```python
from build123d import *

# Parameters (mm, degrees)
SKETCH1_W                     = 312.66
SKETCH1_H                     = 183.16
BODY_DEPTH                    = 4.7
F_6_32_TAPPED_HOLE1_D         = 2.7051
RISER_CABLE_CUTOUT_REACH      = 364.389
EXPANSION_CUTOUT_REACH        = 364.389
SKETCH11_W                    = 138.78
SKETCH11_H                    = 61.66
PSU_CABLE_CUTOUT_REACH        = 364.389
SKETCH20_W                    = 45
SKETCH20_H                    = 15
SSD_ACCESS_CUTOUT_REACH       = 364.389
SKETCH22_W                    = 123.78
SKETCH22_H                    = 72
TAP_DRILL_FOR_M3X0_5_TAP1_D   = 2.5
HOLE_IN_STOCK_REACH           = 364.389
SKETCH33_W                    = 173.88
SKETCH33_H                    = 23.33
BOSS_EXTRUDE1_DEPTH           = 1.5
TAP_DRILL_FOR_6_32_TAP1_D     = 2.7051
TAP_DRILL_FOR_6_32_TAP1_DEPTH = 15.24
TAP_DRILL_FOR_6_32_TAP1_TIP   = 0.81269403
SKETCH32_W                    = 119.186565276
SKETCH32_H                    = 183.16
CUT_EXTRUDE1_DEPTH            = 2


with BuildPart() as part:
    # Sketch1 → body (new body)
    with BuildSketch(Plane(origin=(0, 0, 0), x_dir=(0, 0, -1), z_dir=(1, 0, 0))):
        with Locations((-156.33, 91.58)):
            Rectangle(SKETCH1_W, SKETCH1_H)
    extrude(amount=BODY_DEPTH)

    # #6-32 Tapped Hole1 (through all)
    with Locations(Plane(origin=(4.7, 169.81, 166.8), x_dir=(0, 0, 1), z_dir=(1, 0, 0))):
        with Locations((0, 0), (-154.94, 0), (-132.08, 157.48), (0, 157.48)):
            Hole(F_6_32_TAPPED_HOLE1_D / 2)

    # Sketch8 → riser-cable-cutout (cut, up to next)
    with BuildSketch(Plane(origin=(4.7, 0, 0), x_dir=(0, 0, -1), z_dir=(1, 0, 0)), mode=Mode.PRIVATE) as riser_cable_cutout_sk1:
        Polygon((-148.58070669, 183.16), (-20.810027071, 183.16), (-20.810027071, 176.16), (-20.810027071, 168.16), (-148.58070669, 168.16), (-148.58070669, 176.16), align=None)
    riser_cable_cutout_tool1 = extrude(riser_cable_cutout_sk1.sketch, amount=-RISER_CABLE_CUTOUT_REACH, mode=Mode.PRIVATE) & part.part
    add(riser_cable_cutout_tool1.solids().sort_by_distance((4.7, 175.66, 84.695367))[0], mode=Mode.SUBTRACT)

    # Sketch11 → expansion-cutout (cut, up to next)
    with BuildSketch(Plane(origin=(4.7, 0, 0), x_dir=(0, 0, -1), z_dir=(1, 0, 0)), mode=Mode.PRIVATE) as expansion_cutout_sk1:
        with Locations((-243.27, 30.83)):
            Rectangle(SKETCH11_W, SKETCH11_H)
    expansion_cutout_tool1 = extrude(expansion_cutout_sk1.sketch, amount=-EXPANSION_CUTOUT_REACH, mode=Mode.PRIVATE) & part.part
    add(expansion_cutout_tool1.solids().sort_by_distance((4.7, 30.83, 243.27))[0], mode=Mode.SUBTRACT)

    # Sketch20 → psu-cable-cutout (cut, up to next)
    with BuildSketch(Plane(origin=(4.7, 0, 0), x_dir=(0, 0, -1), z_dir=(1, 0, 0)), mode=Mode.PRIVATE) as psu_cable_cutout_sk1:
        with Locations((-210.16, 175.66)):
            Rectangle(SKETCH20_W, SKETCH20_H)
    psu_cable_cutout_tool1 = extrude(psu_cable_cutout_sk1.sketch, amount=-PSU_CABLE_CUTOUT_REACH, mode=Mode.PRIVATE) & part.part
    add(psu_cable_cutout_tool1.solids().sort_by_distance((4.7, 175.66, 210.16))[0], mode=Mode.SUBTRACT)

    # Sketch22 → ssd-access-cutout (cut, up to next)
    with BuildSketch(Plane(origin=(4.7, 0, 0), x_dir=(0, 0, -1), z_dir=(1, 0, 0)), mode=Mode.PRIVATE) as ssd_access_cutout_sk1:
        with Locations((-240.77, 123.16)):
            Rectangle(SKETCH22_W, SKETCH22_H)
    ssd_access_cutout_tool1 = extrude(ssd_access_cutout_sk1.sketch, amount=-SSD_ACCESS_CUTOUT_REACH, mode=Mode.PRIVATE) & part.part
    add(ssd_access_cutout_tool1.solids().sort_by_distance((4.7, 123.16, 240.77))[0], mode=Mode.SUBTRACT)

    # Tap Drill for M3x0.5 Tap1 (through all)
    with Locations(Plane(origin=(4.7, 0, 0), x_dir=(0, 0, -1), z_dir=(1, 0, 0))):
        with Locations((-298.08, 165.31), (-183.08, 165.31)):
            Hole(TAP_DRILL_FOR_M3X0_5_TAP1_D / 2)

    # Sketch27 → hole-in-stock (cut, up to next)
    with BuildSketch(Plane(origin=(4.7, 0, 0), x_dir=(0, 0, -1), z_dir=(1, 0, 0)), mode=Mode.PRIVATE) as hole_in_stock_sk1:
        with BuildLine():
            Line((0, 114.21), (-84.98, 114.21))
            add(Edge.make_bspline(
                [(-84.98, 114.21), (-62.176533149, 49.839292815), (0, 23.33)],
                knots=[0, 0, 0, 1, 1, 1], degree=2))
            Line((0, 23.33), (0, 114.21))
        make_face()
    hole_in_stock_tool1 = extrude(hole_in_stock_sk1.sketch, amount=-HOLE_IN_STOCK_REACH, mode=Mode.PRIVATE) & part.part
    add(hole_in_stock_tool1.solids().sort_by_distance((4.7, 79.62289, 32.431716))[0], mode=Mode.SUBTRACT)

    # Sketch33 → Boss-Extrude1 (add)
    with BuildSketch(Plane.ZY):
        with Locations((86.94, 11.665)):
            Rectangle(SKETCH33_W, SKETCH33_H)
    extrude(amount=BOSS_EXTRUDE1_DEPTH)

    # Tap Drill for #6-32 Tap1
    with Locations(Plane(origin=(0, 0, 0), x_dir=(-1, 0, 0), z_dir=(0, -1, 0))):
        with Locations((-1.6, -157.446313124), (-1.6, -141.386526913)):
            Hole(TAP_DRILL_FOR_6_32_TAP1_D / 2, depth=TAP_DRILL_FOR_6_32_TAP1_DEPTH)
            with Locations((0, 0, -(TAP_DRILL_FOR_6_32_TAP1_DEPTH + TAP_DRILL_FOR_6_32_TAP1_TIP / 2))):  # 118° drill point
                Cone(0, TAP_DRILL_FOR_6_32_TAP1_D / 2, TAP_DRILL_FOR_6_32_TAP1_TIP, mode=Mode.SUBTRACT)

    # Sketch32 → Cut-Extrude1 (cut)
    with BuildSketch(Plane(origin=(4.7, 0, 0), x_dir=(0, 0, -1), z_dir=(1, 0, 0))):
        with Locations((-100.09076437, 91.58)):
            Rectangle(SKETCH32_W, SKETCH32_H)
    extrude(amount=-CUT_EXTRUDE1_DEPTH, mode=Mode.SUBTRACT)


solid = part.part
```
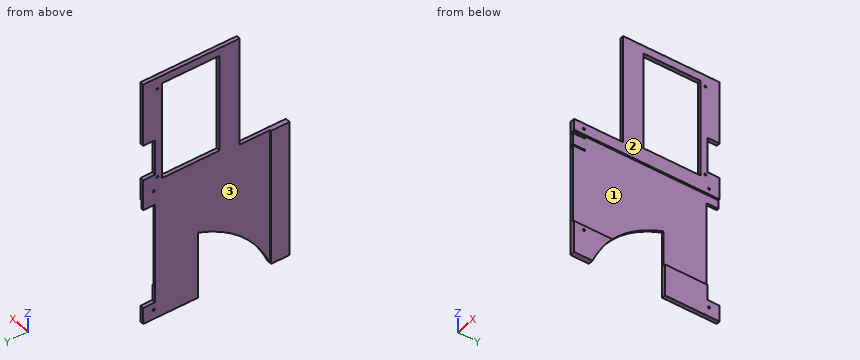
Check sheet for the modelled part. Datum: model origin and axes. Units: mm. Face numbers are marked on the shaded views. A direction names the side the tool comes from. Round coordinates to 2 decimals unless told otherwise and drop trailing zeros. Order: outer loops, then holes, each group sorted by start corner. A loop starts at its lowest first (then second) coordinate and runs counter-clockwise, first axis right, second up. Notation, with made-up numbers: (-4, 63.5) -> (42, 63.5) arc R18 cw to (42, 88.5) -> close; hole circle Ø7 at (5, 79.5). An arc over 180 degrees is marked (long way). One line per item, written item: value. Start each with the question number.
Q1. Cross-section at A-A (z = 207). Record the boundary of the cut face in (x, y).
Q2. Cross-section at B-B (z = 246.5). Record the boundary of the cut face in (x, y), and give its area (3 significant figures).
Q3. Gauge pin test, flat ends, axial feed: pin 1 Ø2 at (x, y) = (2.5, 76.5) entering from -Z; pin 2 Ø4 at (y, z) = (165.31, 183.08) entering from -X; pin 3 Ø3 at (x, y) = (1, 41.5) entering from +Z. Record the tip position at first contact, or that the pin passes through.
Q4. Set-up check for the marked faces 1, 2 and 3: record each of +Z, -Z, +X, -X, +Y, -Y from which the full face is reachable in a straight line by a thin tool's end or side.
Q5. Thickness scan on line 1 (Z direction, x = 2.5, y = 165.31); line 2 (Z direction, x = 3.7, y = 169.81); line 3 (Z direction, x = 1.6, y = 6). Record the ranges inside material, lowest first.
Completed:
1. outline: (0, 61.66) -> (4.7, 61.66) -> (4.7, 87.16) -> (0, 87.16) -> close; (0, 159.16) -> (4.7, 159.16) -> (4.7, 168.16) -> (0, 168.16) -> close
2. outline: (0, 61.66) -> (4.7, 61.66) -> (4.7, 87.16) -> (0, 87.16) -> close; (0, 159.16) -> (4.7, 159.16) -> (4.7, 183.16) -> (0, 183.16) -> close
2. area: 233 mm²
3. pin 1: stops at z = 65.4
3. pin 2: stops at x = 0
3. pin 3: stops at z = 173.88
4. face 1: +X, +Y, -Y
4. face 2: +Z, -Z, +X, +Y, -Y
4. face 3: +Z, -Z, -X, +Y
5. line 1: z = 0 to 181.83, 184.33 to 296.83, 299.33 to 312.66
5. line 2: z = 0 to 10.51, 13.21 to 20.81, 159.68 to 165.45, 168.15 to 187.66, 232.66 to 312.66
5. line 3: z = 0 to 140.03, 142.74 to 156.09, 158.8 to 173.88
